Geometry check sheet. Reference: the model listing, model coordinates, mm. A direction names the side the tool comes from. Coordinates: 2 decimals unless noted, no trailing zeros. Order: outer loops, then holes, each group sorted by start corner. A loop starts at its lowest first (then second) coordinate and runs counter-clockwise, first axis right, second up. Notation, with made-up numbers: M 24,-5.75 L 48,-5.75 A34 cw 48,29.25 Z; hole C -25.5,-23.75 d9. An arc over 180 degrees is marked long. One line per item, written item: value. Start each with the question number.
1) Sectioned sample at A-A, the plane x = 49. Enter the section's corners in (y, z), then the cut area to 3 significant figures.
2) Draft check along X on faces 1 (the cylindrical face through (48.247, 56.104, 49.928)), 2 (the flat face through (56, 64, 47)), 3 (the flat face through (53, 64, 47)), 4 (the flat face through (0, 64, 47)). Enter one of: pulls with the +X half, pulls with the -X half, needs draft (parallel to the pull), parting line crosses it, or undercut.
3) Access from +Z, -Z, +X, -X, +Y, -Y to the whole of each face (thin tool, end or side, straight path). Record for faces 5 (the flat face through (28, 55, 50.942)), 6 (the flat face through (28, 57.976, 50)), 7 (the flat face through (54, 56, 35.648)), 8 (the flat face through (1.479, 79.724, 50.572)), 9 (the flat face through (28, 55, 48.942)).
4) Go/stop test with flat-tipped pins: P1, Ø1.6, axis at x = 27.5, z = 49.5, coming from the +Y side; P2, Ø1.8, axis at x = 31, y = 55.5, coming from the -Z side; P3, Ø3, axis at x = 7, y = 54.92, coming from the +Z side; P4, Ø2, axis at x = 49, y = 54.92, coming from the -Z side. Record where each tip stops, or that it passes through.
5) Sectioned sample at C-C, the plane x = 22. Enter the section's corners in (y, z).
6) Thickness scan on L1, parallel to X at y = 59.5, z = 50; L2, parallel to Y at x = 7, z = 50.05; L3, parallel to Y at x = 39, z = 49.25. Record the ranges inside material, lowest first. Write a range as from..to.
7) Sectioned sample at B-B, the plane z = 37.5. Enter the section's corners in (x, y), then the cut area to 3 significant figures.
```python
from build123d import *

# Parameters (mm, degrees)
EXTRUDE_1_DEPTH     = 3
EXTRUDE_2_DEPTH     = 3
EXTRUDE_3_REACH     = 113.195
SKETCH_5_W          = 2
SKETCH_5_H          = 6
CUT_EXTRUDE_1_REACH = 101.791
SKETCH_8_R          = 1.4


with BuildPart() as part:
    # Sketch 2 → Extrude 1 (new body)
    with BuildSketch(Plane(origin=(0, 0, 0), x_dir=(0, 0, -1), z_dir=(1, 0, 0))):
        Polygon((-47.106132348, 81.520542784), (-35.64838785, 59.42240106), (-35.64838785, 51.976234999), (-53.941911918, 51.976234999), (-53.941911918, 77.976234999), align=None)
    extrude(amount=EXTRUDE_1_DEPTH)


with BuildPart() as body_2:
    # Sketch 3 → Extrude 2 (new body)
    with BuildSketch(Plane(origin=(53, 0, 0), x_dir=(0, 0, -1), z_dir=(1, 0, 0))):
        Polygon((-47.106132348, 81.520542784), (-53.941911918, 77.976234999), (-53.941911918, 51.976234999), (-35.64838785, 51.976234999), (-35.64838785, 59.42240106), align=None)
    extrude(amount=EXTRUDE_2_DEPTH)

    # Sketch 5 → Extrude 3 (add, up to next)
    with BuildSketch(Plane(origin=(3, 0, 0), x_dir=(0, 0, -1), z_dir=(1, 0, 0)), mode=Mode.PRIVATE) as extrude_3_sk1:
        with Locations((-49.941911918, 54.976234999)):
            Rectangle(SKETCH_5_W, SKETCH_5_H)
    extrude_3_tool1 = extrude(extrude_3_sk1.sketch, amount=EXTRUDE_3_REACH, mode=Mode.PRIVATE) - body_2.part

    add(part.part)  # Extrude 3 merges part
    add(extrude_3_tool1.solids().sort_by_distance((3, 54.976235, 49.941912))[0])

    # Sketch 8 → Cut-Extrude 1 (cut, up to next)
    with BuildSketch(Plane(origin=(0, 0, 48.941911918), x_dir=(-1, 0, 0), z_dir=(0, 0, -1)), mode=Mode.PRIVATE) as cut_extrude_1_sk1:
        with Locations((-49, 54.923853845)):
            Circle(SKETCH_8_R)
    cut_extrude_1_tool1 = extrude(cut_extrude_1_sk1.sketch, amount=-CUT_EXTRUDE_1_REACH, mode=Mode.PRIVATE) & body_2.part
    # Sketch 8 → Cut-Extrude 1 (cut, up to next)
    with BuildSketch(Plane(origin=(0, 0, 48.941911918), x_dir=(-1, 0, 0), z_dir=(0, 0, -1)), mode=Mode.PRIVATE) as cut_extrude_1_sk2:
        with Locations((-7, 54.923853845)):
            Circle(SKETCH_8_R)
    cut_extrude_1_tool2 = extrude(cut_extrude_1_sk2.sketch, amount=-CUT_EXTRUDE_1_REACH, mode=Mode.PRIVATE) & body_2.part
    add(cut_extrude_1_tool1.solids().sort_by_distance((49, 54.923854, 48.941912))[0], mode=Mode.SUBTRACT)
    add(cut_extrude_1_tool2.solids().sort_by_distance((7, 54.923854, 48.941912))[0], mode=Mode.SUBTRACT)


solid = body_2.part
```
Final values:
1. outline: M 51.98,48.94 L 53.52,48.94 L 53.52,50.94 L 51.98,50.94 Z; M 56.32,48.94 L 57.98,48.94 L 57.98,50.94 L 56.32,50.94 Z
1. area: 6.40 mm^2
2. face 1: undercut
2. face 2: pulls with the +X half
2. face 3: undercut
2. face 4: pulls with the -X half
3. face 5: +Z, +Y, -Y
3. face 6: +Z, -Z, +Y
3. face 7: -Z, +X, -X, +Y, -Y
3. face 8: +Z, +X, -X, +Y
3. face 9: -Z, +Y, -Y
4. P1: stops at y = 57.98
4. P2: stops at z = 48.94
4. P3: stops at z = 50.94
4. P4: passes through
5. outline: M 51.98,48.94 L 57.98,48.94 L 57.98,50.94 L 51.98,50.94 Z
6. L1: x = 0..3, 53..56
6. L2: y = 51.98..53.52, 56.32..57.98
6. L3: y = 51.98..57.98
7. outline: M 0,51.98 L 3,51.98 L 3,62.99 L 0,62.99 Z; M 53,51.98 L 56,51.98 L 56,62.99 L 53,62.99 Z
7. area: 66.1 mm^2
